from build123d import *

# Parameters (mm, degrees)
EXTRUDE_1_DEPTH = 5
SKETCH_2_R      = 1.4
EXTRUDE_2_DEPTH = 3


with BuildPart() as part:
    # 草图1 → 凸台-拉伸1 (new body)
    with BuildSketch(Plane.XY):
        with BuildLine():
            Line((-45, 0), (-40, 0))
            ThreePointArc((-40, 0), (0, 40), (40, 0))
            Line((40, 0), (45, 0))
            ThreePointArc((45, 0), (0, 45), (-45, 0))
        make_face()
    extrude(amount=EXTRUDE_1_DEPTH)

    # 草图2 → 凸台-拉伸2 (add)
    with BuildSketch(Plane.XZ):
        with BuildLine():
            Line((-45, 5), (-50, 5))
            ThreePointArc((-50, 5), (-52.5, 2.5), (-50, 0))
            Line((-50, 0), (-45, 0))
            Line((-45, 0), (-44.132295493, 0))
            Line((-44.132295493, 0), (-44.132295493, 5))
            Line((-44.132295493, 5), (-45, 5))
        make_face()
        with Locations((-50, 2.5)):
            Circle(SKETCH_2_R, mode=Mode.SUBTRACT)
        with BuildLine():
            Line((44.132295493, 5), (44.132295493, 0))
            Line((44.132295493, 0), (45, 0))
            Line((45, 0), (50, 0))
            ThreePointArc((50, 0), (52.5, 2.5), (50, 5))
            Line((50, 5), (45, 5))
            Line((45, 5), (44.132295493, 5))
        make_face()
        with Locations((50, 2.5)):
            Circle(SKETCH_2_R, mode=Mode.SUBTRACT)
    extrude(amount=-EXTRUDE_2_DEPTH)


solid = part.part
Geometry check sheet. Reference: the model listing, model coordinates, mm. A direction names the side the tool comes from. Round coordinates to 2 decimals unless told otherwise and drop trailing zeros. Order: outer loops, then holes, each group sorted by start corner. A loop starts at its lowest first (then second) coordinate and runs counter-clockwise, first axis right, second up. Notation, with made-up numbers: M 65.25,-1.5 L 98.25,-1.5 A25 ccw 98.25,12.5 Z; hole C 1,-25 d8. An arc over 180 degrees is marked long. Answer in a Markdown table with one row per item. Add a question column.
Item 1: Draft check along X on faces 4 (the face through (52.5, 1.5, 2.4)), 5 (the face through (-45, 0, 3)), 6 (the face through (-48.71, 1.48, 1.96)). Enter one of: released by +X, released by -X, zero draft, split by the parting line, or undercut.
Item 2: Sectioned sample at D-D, the plane y = 37. Enter the section's corners in (x, z), plus the area to 3 significant figures.
Item 3: Depth check by flat-ended pin: pin 1 Ø2 at (x, z) = (-35, 1.5) entering from +Y; pin 2 Ø3 at (y, z) = (16.5, 4.5) entering from -X; pin 3 Ø1.5 at (x, z) = (48.5, 2.5) entering from +Y. Enter the tip coordinate at first touch or a pass-through.
Item 4: Sectioned sample at A-A, the plane z = 2.5. Enter the section's corners in (x, y), plus the area to 3 significant figures.
Item 5: Sectioned sample at C-C, the plane x = 0. Enter the section's corners in (y, z).
Item 6: Sectioned sample at B-B, the plane y = 28. Enter the section's corners in (x, z).
Item 7: Material ranges on L1, parallel to Z at x = -50, y = 1.6; L2, parallel to X at y = 27.5, z = 1.95; L3, parallel to X at y = 9, z = 4.5, recorded low to high. Write a range as [from, to].
Item 8: Set-up check for faces 1 (the face through (-48, 3, 3)), 2 (the face through (48, 3, 3)), 3 (the face through (0, 41, 0)): record each of +Z, -Z, +X, -X, +Y, -Y from which the full face is reachable in a straight line by a thin tool's end or side.
Filled in:
| question | item | result |
|---|---|---|
| 1 | face 4 | released by +X |
| 1 | face 5 | zero draft |
| 1 | face 6 | undercut |
| 2 | outline | M -25.61,0 L -15.2,0 L -15.2,5 L -25.61,5 Z; M 15.2,0 L 25.61,0 L 25.61,5 L 15.2,5 Z |
| 2 | area | 104 mm² |
| 3 | pin 1 | stops at y = 29.48 |
| 3 | pin 2 | stops at x = -42.43 |
| 3 | pin 3 | stops at y = 3 |
| 4 | outline | M -52.5,0 L -51.4,0 L -51.4,3 L -52.5,3 Z; M -48.6,0 L -40,0 A40 cw 40,0 L 48.6,0 L 48.6,3 L 44.9,3 A45 ccw -44.9,3 L -48.6,3 Z; M 51.4,0 L 52.5,0 L 52.5,3 L 51.4,3 Z |
| 4 | area | 696 mm² |
| 5 | outline | M 40,0 L 45,0 L 45,5 L 40,5 Z |
| 6 | outline | M -35.23,0 L -28.57,0 L -28.57,5 L -35.23,5 Z; M 28.57,0 L 35.23,0 L 35.23,5 L 28.57,5 Z |
| 7 | L1 | z = [0, 1.1], [3.9, 5] |
| 7 | L2 | x = [-35.62, -29.05], [29.05, 35.62] |
| 7 | L3 | x = [-44.09, -38.97], [38.97, 44.09] |
| 8 | face 1 | +Z, -Z, -X, +Y |
| 8 | face 2 | +Z, -Z, +X, +Y |
| 8 | face 3 | -Z, +X, -X, +Y, -Y |
